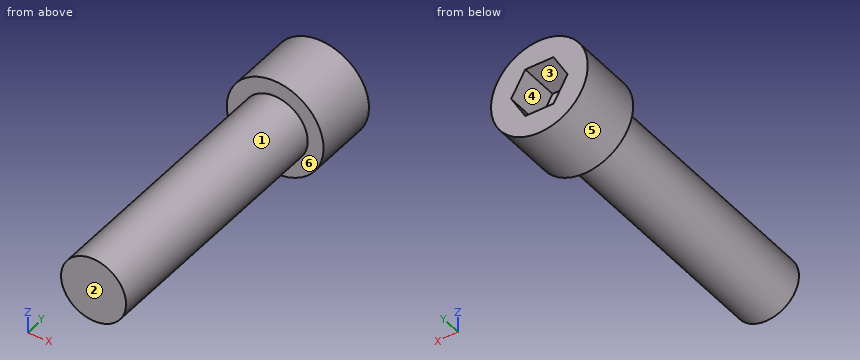
```python
from build123d import *

# Parameters (mm, degrees)
HEX_CUT_DEPTH = 3.81


with BuildPart() as part:
    # Sketch1 → Screw revolve (revolve)
    with BuildSketch(Plane.XY, mode=Mode.PRIVATE) as screw_revolve_sk:
        Polygon((0, 0), (3.175, 0), (3.175, 25.4), (4.7244, 25.4), (4.7244, 31.75), (0, 31.75), align=None)
    revolve(screw_revolve_sk.sketch.rotate(Axis((0, 0, 0), (0, 1, 0)), 90), axis=Axis((0, 0, 0), (0, 1, 0)))

    # Sketch2 → Hex Cut (cut)
    with BuildSketch(Plane(origin=(0, 31.75, 0), x_dir=(-1, 0, 0), z_dir=(0, 1, 0))):
        Polygon((-2.756963005, 0), (-1.378481503, -2.3876), (1.378481503, -2.3876), (2.756963005, 0), (1.378481503, 2.3876), (-1.378481503, 2.3876), align=None)
    extrude(amount=-HEX_CUT_DEPTH, mode=Mode.SUBTRACT)


solid = part.part
```
The model under review builds one solid part; all positions refer to its coordinate system, in mm. Face numbers are marked on the shaded views. A direction names the side the tool comes from. Round coordinates to 2 decimals unless told otherwise and drop trailing zeros. Loops run counter-clockwise (first coordinate to the right, second up) from the corner with the lowest first, then second, coordinate; pieces in that order, holes last. Notation, with made-up numbers: (-0.75, 14) - (39.25, 14) arc R14 cw to (39.25, 40) - close; hole circle Ø3 at (18.25, 31). An arc over 180 degrees is marked (long way). Write each question's results on one line, items separated by ' | '. Start each with the question number.
Q1. Tool access review of the marked faces 1 and 2: name each direction out of +Z, -Z, +X, -X, +Y, -Y from which nothing blocks a thin tool from reaching the whole face with its end or side.
Q2. Wall thickness on line 1 along X through (y, z) = (26, 3.5); line 2 along Y through (x, z) = (0, 4); line 3 along Z through (x, y) = (-2.5, 28.5): over which ranges is each line inside the solid? List them lowest first. Write a range as [from, to].
Q3. Take a section at B-B on y = 17.5. Give the boundary of the cut face in (x, z) (3 decimals), plus the area to 3 significant figures.
Q4. Draft analysis for pull direction Z (two halves, no side actions). For the marked faces 3, 4, 5 and 6, state which applies: pulls with the +Z half, pulls with the -Z half, needs draft (parallel to the pull), parting line crosses it, or undercut.
Q5. Take a section at A-A on x = 0. Give the boundary of the cut face in (y, z) (3 decimals).
Q6. Insertion check: P1, Ø1, axis at x = -1.5, z = -1.5, coming from the +Y side; P2, Ø1, axis at y = 7.5, z = 1.5, coming from the -X side; P3, Ø4, axis at x = 2.5, y = 6, coming from the -Z side; P4, Ø3, axis at y = 17, z = 1.5, coming from the -X side (3 decimals). Each pin has a flat end and moves straight along its axis. Give the tip position at first contact, or say it passes through.
Data:
1) face 1: -Y | face 2: +Z, -Z, +X, -X, -Y
2) line 1: x = [-3.17, 3.17] | line 2: y = [25.4, 31.75] | line 3: z = [-4.01, -0.45], [0.45, 4.01]
3) outline: circle Ø6.35 at (0, 0) | area: 31.7 mm²
4) face 3: undercut | face 4: undercut | face 5: parting line crosses it | face 6: needs draft
5) outline: (0, -3.175) - (25.4, -3.175) - (25.4, -4.724) - (31.75, -4.724) - (31.75, -2.388) - (27.94, -2.388) - (27.94, 2.388) - (31.75, 2.388) - (31.75, 4.724) - (25.4, 4.724) - (25.4, 3.175) - (0, 3.175) - close
6) P1: stops at y = 31.75 | P2: stops at x = -3.01 | P3: stops at z = -3.14 | P4: stops at x = -3.175
